from build123d import *

# Parameters (mm, degrees)
SKETCH_1_W           = 250
SKETCH_1_H           = 29
SKETCH_1_W_2         = 30
SKETCH_1_H_2         = 15
EXTRUDE_1_DEPTH      = 28
SKETCH_1_3_R         = 2
CUT_EXTRUDE_1_DEPTH  = 132.450561049
CUT_EXTRUDE_START    = 2
SKETCH_1_5_R         = 2
CUT_EXTRUDE_2_DEPTH  = 24
SKETCH_3_W           = 6
SKETCH_3_H           = 19
EXTRUDE_2_DEPTH      = 35
SKETCH_3_3_W         = 6
SKETCH_3_3_H         = 19
EXTRUDE_3_DEPTH      = 35
SKETCH_1_6_R         = 2
CUT_EXTRUDE_3_DEPTH  = 166.088612569
CUT_EXTRUDE_7_REACH  = 167.089
SKETCH_1_8_R         = 2.6
FILLET_1_R           = 9.5
FILLET_2_R           = 5
SKETCH_4_R           = 5.1
CUT_EXTRUDE_4_DEPTH  = 31.5
SKETCH_4_2_OUTSIDE_W = 87.946
SKETCH_4_2_OUTSIDE_H = 103.946
SKETCH_4_2_OUTSIDE_R = 5.1
CUT_EXTRUDE_5_DEPTH  = 21.5
SKETCH_5_OUTSIDE_W   = 83.722
SKETCH_5_OUTSIDE_H   = 99.722
SKETCH_5_OUTSIDE_W_2 = 23.8
SKETCH_5_OUTSIDE_H_2 = 24.8
CUT_EXTRUDE_6_DEPTH  = 18


with BuildPart() as part:
    # 草图1 → 凸台-拉伸1 (new body)
    with BuildSketch(Plane(origin=(0, 0, 0), x_dir=(0, 0, -1), z_dir=(1, 0, 0))):
        Rectangle(SKETCH_1_W, SKETCH_1_H)
        with Locations((-60, 22)):
            Rectangle(SKETCH_1_W_2, SKETCH_1_H_2)
        with Locations((0, 22)):
            Rectangle(SKETCH_1_W_2, SKETCH_1_H_2)
        with Locations((60, 22)):
            Rectangle(SKETCH_1_W_2, SKETCH_1_H_2)
    extrude(amount=EXTRUDE_1_DEPTH)

    # 草图1<3> → 切除-拉伸1 (cut, through all)
    with BuildSketch(Plane(origin=(0, 0, 0), x_dir=(0, 0, -1), z_dir=(1, 0, 0))):
        with Locations((-67.5, -10.858617882)):
            Circle(SKETCH_1_3_R)
        with Locations((-22.5, -10.858617882)):
            Circle(SKETCH_1_3_R)
        with Locations((22.5, -10.858617882)):
            Circle(SKETCH_1_3_R)
        with Locations((-60, 25.5)):
            Circle(SKETCH_1_3_R)
        with Locations((67.5, -10.858617882)):
            Circle(SKETCH_1_3_R)
        with Locations((0, 25.5)):
            Circle(SKETCH_1_3_R)
        with Locations((60, 25.5)):
            Circle(SKETCH_1_3_R)
    extrude(amount=CUT_EXTRUDE_1_DEPTH, mode=Mode.SUBTRACT)

    # 草图1<5> → 切除-拉伸2 (cut)
    # profile 1 of 7: a face of its own
    with BuildSketch(Plane(origin=(0, 0, 0), x_dir=(0, 0, -1), z_dir=(1, 0, 0)).offset(CUT_EXTRUDE_START)):
        with BuildLine():
            Line((-72.5, 29.5), (-72.5, 25.5))
            ThreePointArc((-72.5, 25.5), (-60, 13), (-47.5, 25.5))
            Line((-47.5, 25.5), (-47.5, 29.5))
            Line((-47.5, 29.5), (-72.5, 29.5))
        make_face()
        with Locations((-60, 25.5)):
            Circle(SKETCH_1_5_R, mode=Mode.SUBTRACT)
    # profile 2 of 7: a face of its own
    with BuildSketch(Plane(origin=(0, 0, 0), x_dir=(0, 0, -1), z_dir=(1, 0, 0)).offset(CUT_EXTRUDE_START)):
        with BuildLine():
            Line((-79.457856675, -14.5), (-55.542143325, -14.5))
            ThreePointArc((-55.542143325, -14.5), (-67.5, 1.641382118), (-79.457856675, -14.5))
        make_face()
        with Locations((-67.5, -10.858617882)):
            Circle(SKETCH_1_5_R, mode=Mode.SUBTRACT)
    # profile 3 of 7: a face of its own
    with BuildSketch(Plane(origin=(0, 0, 0), x_dir=(0, 0, -1), z_dir=(1, 0, 0)).offset(CUT_EXTRUDE_START)):
        with BuildLine():
            Line((-34.457856675, -14.5), (-10.542143325, -14.5))
            ThreePointArc((-10.542143325, -14.5), (-22.5, 1.641382118), (-34.457856675, -14.5))
        make_face()
        with Locations((-22.5, -10.858617882)):
            Circle(SKETCH_1_5_R, mode=Mode.SUBTRACT)
    # profile 4 of 7: a face of its own
    with BuildSketch(Plane(origin=(0, 0, 0), x_dir=(0, 0, -1), z_dir=(1, 0, 0)).offset(CUT_EXTRUDE_START)):
        with BuildLine():
            ThreePointArc((-12.5, 25.5), (0, 13), (12.5, 25.5))
            Line((12.5, 25.5), (12.5, 29.5))
            Line((12.5, 29.5), (-12.5, 29.5))
            Line((-12.5, 29.5), (-12.5, 25.5))
        make_face()
        with Locations((0, 25.5)):
            Circle(SKETCH_1_5_R, mode=Mode.SUBTRACT)
    # profile 5 of 7: a face of its own
    with BuildSketch(Plane(origin=(0, 0, 0), x_dir=(0, 0, -1), z_dir=(1, 0, 0)).offset(CUT_EXTRUDE_START)):
        with BuildLine():
            Line((10.542143325, -14.5), (34.457856675, -14.5))
            ThreePointArc((34.457856675, -14.5), (22.5, 1.641382118), (10.542143325, -14.5))
        make_face()
        with Locations((22.5, -10.858617882)):
            Circle(SKETCH_1_5_R, mode=Mode.SUBTRACT)
    # profile 6 of 7: a face of its own
    with BuildSketch(Plane(origin=(0, 0, 0), x_dir=(0, 0, -1), z_dir=(1, 0, 0)).offset(CUT_EXTRUDE_START)):
        with BuildLine():
            Line((55.542143325, -14.5), (79.457856675, -14.5))
            ThreePointArc((79.457856675, -14.5), (67.5, 1.641382118), (55.542143325, -14.5))
        make_face()
        with Locations((67.5, -10.858617882)):
            Circle(SKETCH_1_5_R, mode=Mode.SUBTRACT)
    # profile 7 of 7: a face of its own
    with BuildSketch(Plane(origin=(0, 0, 0), x_dir=(0, 0, -1), z_dir=(1, 0, 0)).offset(CUT_EXTRUDE_START)):
        with BuildLine():
            ThreePointArc((47.5, 25.5), (60, 13), (72.5, 25.5))
            Line((72.5, 25.5), (72.5, 29.5))
            Line((72.5, 29.5), (47.5, 29.5))
            Line((47.5, 29.5), (47.5, 25.5))
        make_face()
        with Locations((60, 25.5)):
            Circle(SKETCH_1_5_R, mode=Mode.SUBTRACT)
    extrude(amount=CUT_EXTRUDE_2_DEPTH, mode=Mode.SUBTRACT)

    # 草图3 → 凸台-拉伸2 (add)
    with BuildSketch(Plane.XY.offset(125)):
        with Locations((25, 0)):
            Rectangle(SKETCH_3_W, SKETCH_3_H)
    extrude(amount=EXTRUDE_2_DEPTH)

    # 草图3<3> → 凸台-拉伸3 (add)
    with BuildSketch(Plane.XY.offset(125)):
        with Locations((25, 0)):
            Rectangle(SKETCH_3_3_W, SKETCH_3_3_H)
        with Locations((3, 0)):
            Rectangle(SKETCH_3_3_W, SKETCH_3_3_H)
    extrude(amount=EXTRUDE_3_DEPTH)

    # 草图1<6> → 切除-拉伸3 (cut, through all)
    with BuildSketch(Plane(origin=(0, 0, 0), x_dir=(0, 0, -1), z_dir=(1, 0, 0))):
        with Locations(Location((-150, 0, 0), (0, 0, 90))):
            Circle(SKETCH_1_6_R)
    extrude(amount=CUT_EXTRUDE_3_DEPTH, mode=Mode.SUBTRACT)

    # 草图1<8> → 切除-拉伸7 (cut, up to next)
    with BuildSketch(Plane(origin=(0, 0, 0), x_dir=(0, 0, -1), z_dir=(1, 0, 0)), mode=Mode.PRIVATE) as cut_extrude_7_sk1:
        with Locations(Location((-150, 0, 0), (0, 0, 180))):
            Circle(SKETCH_1_8_R)
    cut_extrude_7_tool1 = extrude(cut_extrude_7_sk1.sketch, amount=CUT_EXTRUDE_7_REACH, mode=Mode.PRIVATE) & part.part
    add(cut_extrude_7_tool1.solids().sort_by_distance((0, 0, 150))[0], mode=Mode.SUBTRACT)

    # 圆角1
    fillet_1_edges = [part.edges().sort_by_distance(p)[0] for p in [
        (25, 9.5, 160),
        (25, -9.5, 160),
        (3, -9.5, 160),
        (3, 9.5, 160),
    ]]
    fillet(fillet_1_edges, radius=FILLET_1_R - 0.0001)  # a hair under: the kernel refuses the full size

    # 圆角2
    fillet_2_edges = [part.edges().sort_by_distance(p)[0] for p in [
        (14, -14.5, 125),
        (14, 14.5, 125),
    ]]
    fillet(fillet_2_edges, radius=FILLET_2_R)

    # 草图4 → 切除-拉伸4 (cut)
    with BuildSketch(Plane(origin=(0, 0, -125), x_dir=(-1, 0, 0), z_dir=(0, 0, -1))):
        with Locations((-14, 0)):
            Circle(SKETCH_4_R)
    extrude(amount=-CUT_EXTRUDE_4_DEPTH, mode=Mode.SUBTRACT)

    # 草图4<2> outside → 切除-拉伸5 (cut)
    with BuildSketch(Plane(origin=(0, 0, -125), x_dir=(-1, 0, 0), z_dir=(0, 0, -1))):
        with Locations((-14, 7.5)):
            Rectangle(SKETCH_4_2_OUTSIDE_W, SKETCH_4_2_OUTSIDE_H)
        with Locations((-14, 0)):
            Circle(SKETCH_4_2_OUTSIDE_R, mode=Mode.SUBTRACT)
    extrude(amount=-CUT_EXTRUDE_5_DEPTH, mode=Mode.SUBTRACT)

    # 草图5 outside → 切除-拉伸6 (cut)
    with BuildSketch(Plane(origin=(0, 0, -103.5), x_dir=(-1, 0, 0), z_dir=(0, 0, -1))):
        with Locations((-14, 7.5)):
            Rectangle(SKETCH_5_OUTSIDE_W, SKETCH_5_OUTSIDE_H)
        with Locations((-14, 0)):
            Rectangle(SKETCH_5_OUTSIDE_W_2, SKETCH_5_OUTSIDE_H_2, mode=Mode.SUBTRACT)
    extrude(amount=-CUT_EXTRUDE_6_DEPTH, mode=Mode.SUBTRACT)


solid = part.part
Part model, mm, in its own coordinate system. A direction names the side the tool comes from. Coordinates: 2 decimals unless noted, no trailing zeros. Write each loop counter-clockwise with the first axis right and the second up, starting at its lowest first coordinate (ties: lowest second). Pieces come first, ordered by that corner, then holes. Notation, with made-up numbers: (-27.75, 5) - (-20.75, 5) arc R26 ccw to (-20.75, 26) - close; hole circle Ø8 at (41, 13.5). An arc over 180 degrees is marked (long way). Put each result on its own line as item: value.
1. Probe line 1 along Z through (x, y) = (27.35, 25.5); line 2 along Z through (x, y) = (4, 15.5); line 3 along Y through (x, z) = (27.5, 22.5). List the from-to ranges inside material, lowest first. Write a range as [from, to].
Final values:
line 1: z = [-75, -62], [-58, -45], [-15, -2], [2, 15], [45, 58], [62, 75]
line 2: z = [-75, -67.5], [-52.5, -45], [-15, -7.5], [7.5, 15], [45, 52.5], [67.5, 75]
line 3: y = [-14.5, -12.86], [-8.86, 14.5]
2. Band-saw the part on A-A (y = 18). Write the cut outline in (x, z).
Final values:
outline: (0, -75) - (28, -75) - (28, -45) - (0, -45) - close; (0, -15) - (28, -15) - (28, 15) - (0, 15) - close; (0, 45) - (28, 45) - (28, 75) - (0, 75) - close; hole (2, -70) - (26, -70) - (26, -50) - (2, -50) - close; hole (2, -10) - (26, -10) - (26, 10) - (2, 10) - close; hole (2, 50) - (26, 50) - (26, 70) - (2, 70) - close
3. Two-plate mould, pull along Z, no slides. Class faces 5 (the flat face through (26, 23, -60)), 6 (the cylindrical face through (25.042, 6.643, 157.291)), 7 (the flat face through (22, 0, 142)): +Z half, -Z half, draft (parallel to the pull), parting line (faces both ways), or undercut.
Final values:
face 5: undercut
face 6: +Z half
face 7: draft
4. Band-saw the part on B-B (z = 18). Write the cut outline in (x, y), then the cut area to 3 significant figures.
Final values:
outline: (0, -14.5) - (2, -14.5) - (2, 0.8) - (26, 0.8) - (26, -14.5) - (28, -14.5) - (28, 14.5) - (0, 14.5) - close
area: 445 mm²
5. 3-axis set-ups, long thin cutter, end or side, ignore diameter. For faces 1 (the flat face through (14, 14.5, -30)), 2 (the flat face through (6, 0, 142)), 3 (the flat face through (26, 23, 60)), 4 (the flat face through (25.9, 0, -95)): which of +Z, -Z, +X, -X, +Y, -Y reach the whole face in a straight line?
Final values:
face 1: +X, -X, +Y
face 2: +Z, +Y, -Y
face 3: +Y
face 4: -Z, +X, +Y, -Y
6. Flat gauge pins, fed straight in: pin 1 Ø14.5 at (y, z) = (5, -96) entering from -X; pin 2 Ø1.5 at (x, y) = (8, 2) entering from +Z; pin 3 Ø4.5 at (x, y) = (11.5, 19.5) entering from +Z; pin 4 Ø13 at (y, z) = (-5, 21) entering from -X. Where does each tip first touch, or does it go through?
Final values:
pin 1: stops at x = 2.1
pin 2: stops at z = 125
pin 3: stops at z = 75
pin 4: stops at x = 0
